```python
from build123d import *

# Parameters (mm, degrees)
F1_DEPTH = 12
F0_R     = 1.5
F2_DEPTH = 3
F4_DEPTH = 6
F5_W     = 20.872174
F5_H     = 2.650432
F5_W_2   = 2.650432
F5_H_2   = 20.872174
F6_DEPTH = 9.001


with BuildPart() as f1:
    # F0 (on Top) → F1 (new body)
    with BuildSketch(Plane.XY):
        Polygon((36.522065, 27.258966), (27.188256, 17.925157), (17.925157, 27.188256), (27.258966, 36.522065), (30.258966, 39.522065), (27.258966, 39.522065), (0, 39.522065), (-27.258966, 39.522065), (-30.258966, 39.522065), (-27.258966, 36.522065), (-17.925157, 27.188256), (-27.188256, 17.925157), (-36.522065, 27.258966), (-39.522065, 30.258966), (-39.522065, 27.258966), (-39.522065, 0), (-39.522065, -27.258966), (-39.522065, -30.258966), (-36.522065, -27.258966), (-27.188256, -17.925157), (-17.925157, -27.188256), (-27.258966, -36.522065), (-30.258966, -39.522065), (-27.258966, -39.522065), (0, -39.522065), (27.258966, -39.522065), (30.258966, -39.522065), (27.258966, -36.522065), (17.925157, -27.188256), (27.188256, -17.925157), (36.522065, -27.258966), (39.522065, -30.258966), (39.522065, -27.258966), (39.522065, 0), (39.522065, 27.258966), (39.522065, 30.258966), align=None)
    extrude(amount=F1_DEPTH)

    # F0 (on Top) + F1_face (on face) → F2 (join)
    with BuildSketch(Plane.XY):
        Polygon((-31.501607, -39.522065), (-30.258966, -39.522065), (-27.258966, -36.522065), (-17.925157, -27.188256), (-27.188256, -17.925157), (-36.522065, -27.258966), (-39.522065, -30.258966), (-39.522065, -31.501607), align=None)
        with Locations((-31.041988, -31.041988)):
            Circle(F0_R, mode=Mode.SUBTRACT)
        with Locations((-25.385133, -25.385133)):
            Circle(F0_R, mode=Mode.SUBTRACT)
        Polygon((-27.258966, 36.522065), (-30.258966, 39.522065), (-31.501607, 39.522065), (-39.522065, 31.501607), (-39.522065, 30.258966), (-36.522065, 27.258966), (-27.188256, 17.925157), (-17.925157, 27.188256), align=None)
        with Locations((-25.385133, 25.385133)):
            Circle(F0_R, mode=Mode.SUBTRACT)
        with Locations((-31.041988, 31.041988)):
            Circle(F0_R, mode=Mode.SUBTRACT)
        Polygon((17.925157, 27.188256), (27.188256, 17.925157), (36.522065, 27.258966), (39.522065, 30.258966), (39.522065, 31.501607), (31.501607, 39.522065), (30.258966, 39.522065), (27.258966, 36.522065), align=None)
        with Locations((25.385133, 25.385133)):
            Circle(F0_R, mode=Mode.SUBTRACT)
        with Locations((31.041988, 31.041988)):
            Circle(F0_R, mode=Mode.SUBTRACT)
        Polygon((39.522065, -31.501607), (39.522065, -30.258966), (36.522065, -27.258966), (27.188256, -17.925157), (17.925157, -27.188256), (27.258966, -36.522065), (30.258966, -39.522065), (31.501607, -39.522065), align=None)
        with Locations((31.041988, -31.041988)):
            Circle(F0_R, mode=Mode.SUBTRACT)
        with Locations((25.385133, -25.385133)):
            Circle(F0_R, mode=Mode.SUBTRACT)
    with BuildSketch(Plane.XY.offset(12)):
        Polygon((27.188256, -17.925157), (39.522065, -30.258966), (39.522065, 30.258966), (27.188256, 17.925157), (17.925157, 27.188256), (30.258966, 39.522065), (-30.258966, 39.522065), (-17.925157, 27.188256), (-27.188256, 17.925157), (-39.522065, 30.258966), (-39.522065, -30.258966), (-27.188256, -17.925157), (-17.925157, -27.188256), (-30.258966, -39.522065), (30.258966, -39.522065), (17.925157, -27.188256), align=None)
    extrude(amount=F2_DEPTH)

    # F3 (on face) → F4 (cut)
    with BuildSketch(Plane.XY.offset(15)):
        Polygon((-26.016326, 39.522065), (-13.682516, 27.188256), (13.682516, 27.188256), (26.016326, 39.522065), align=None)
        Polygon((13.682516, 27.188256), (-13.682516, 27.188256), (-27.188256, 13.682516), (-27.188256, 0), (-27.188256, -13.682516), (-13.682516, -27.188256), (13.682516, -27.188256), (27.188256, -13.682516), (27.188256, 0), (27.188256, 13.682516), align=None)
        Polygon((-27.188256, 0), (-27.188256, 13.682516), (-39.522065, 26.016326), (-39.522065, 0), (-39.522065, -26.016326), (-27.188256, -13.682516), align=None)
        Polygon((39.522065, 26.016326), (27.188256, 13.682516), (27.188256, 0), (27.188256, -13.682516), (39.522065, -26.016326), (39.522065, 0), align=None)
        Polygon((13.682516, -27.188256), (-13.682516, -27.188256), (-26.016326, -39.522065), (26.016326, -39.522065), align=None)
    extrude(amount=-F4_DEPTH, mode=Mode.SUBTRACT)

    # F5 (on face) → F6 (cut, through all)
    with BuildSketch(Plane.XY.offset(9)):
        with Locations((0, 31.473912)):
            Rectangle(F5_W, F5_H)
        with Locations((-31.473912, 0)):
            Rectangle(F5_W_2, F5_H_2)
        with Locations((0, -31.473912)):
            Rectangle(F5_W, F5_H)
        with Locations((31.473912, 0)):
            Rectangle(F5_W_2, F5_H_2)
    extrude(amount=-F6_DEPTH, mode=Mode.SUBTRACT)


solid = f1.part
```
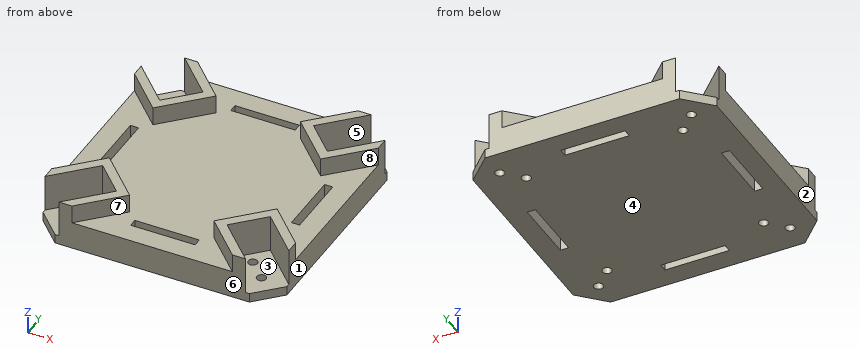
Check sheet for the modelled part. Datum: model origin and axes. Units: mm. Face numbers are marked on the shaded views. A direction names the side the tool comes from. Round coordinates to 2 decimals unless told otherwise and drop trailing zeros. Loops run counter-clockwise (first coordinate to the right, second up) from the corner with the lowest first, then second, coordinate; pieces in that order, holes last. Notation, with made-up numbers: (12.25, 12.25) - (37.25, 12.25) arc R31 cw to (37.25, 37.25) - close; hole circle Ø1 at (52.25, 28). An arc over 180 degrees is marked (long way). Answer as a JSON object with one key per item and string values. Group by question number.
Q1. Sectioned sample at A-A, the plane x = -1. Enter the section's corners in (y, z).
Q2. Scan lines: line 1 along Y through (x, z) = (-5.5, 6); line 2 along Y through (x, z) = (24, 11). Record each from-to range of solid material in increasing order. Write a range as [from, to].
Q3. Set-up check for the marked faces 5, 6, 7 and 8: record each of +Z, -Z, +X, -X, +Y, -Y from which the full face is reachable in a straight line by a thin tool's end or side.
Q4. Mould release check, pull along X, two halves, no side actions. Record for the marked faces 1, 2, 3 and 4: released by +X, released by -X, zero draft, split by the parting line, or undercut.
Q5. Sectioned sample at C-C, the plane z = 12. Count the separate pieces of the cut face and the enclosed holes in it, plus the area to 3 significant figures.
Q6. Gauge pin test, flat ends, axial feed: P1, Ø2, axis at y = 17, z = 12.5, coming from the +X side; P2, Ø12, axis at x = -0.5, y = 6.5, coming from the +Z side; P3, Ø2, axis at x = -31.5, z = 5.5, coming from the +Y side. Record the tip position at first contact, or that the pin passes through.
Solution:
{
 "1": {"outline": "(-39.52, 0) - (-32.8, 0) - (-32.8, 9) - (-39.52, 9) - close; (-30.15, 0) - (30.15, 0) - (30.15, 9) - (-30.15, 9) - close; (32.8, 0) - (39.52, 0) - (39.52, 9) - (32.8, 9) - close"},
 "2": {"line 1": "y = [-39.52, -32.8], [-30.15, 30.15], [32.8, 39.52]", "line 2": "y = [-37.51, -33.26], [-21.11, -16.87], [16.87, 21.11], [33.26, 37.51]"},
 "3": {"face 5": "+Z", "face 6": "+Z, -Z, +X, -X, -Y", "face 7": "+Z, -Y", "face 8": "+Z, +X"},
 "4": {"face 1": "released by +X", "face 2": "released by -X", "face 3": "undercut", "face 4": "zero draft"},
 "5": {"separate pieces": "4", "enclosed holes": "0", "area": "612 mm²"},
 "6": {"P1": "stops at x = 31.51", "P2": "stops at z = 9", "P3": "stops at y = 23.24"}
}
